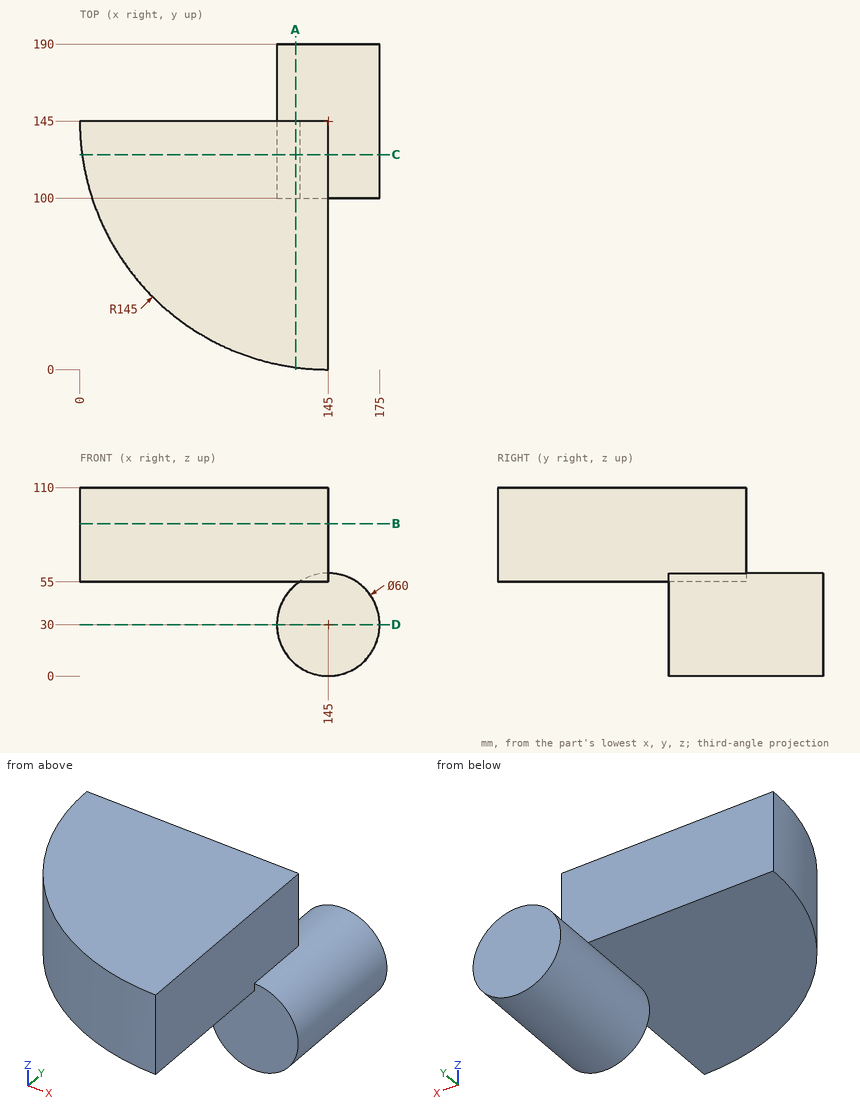
Part print with two shaded views. Sizes in mm from the minimum x, y, z corner. Coordinates: 2 decimals unless noted, no trailing zeros. Write each loop counter-clockwise with the first axis right and the second up, starting at its lowest first coordinate (ties: lowest second). Pieces come first, ordered by that corner, then holes. Notation, with made-up numbers: M -30,65.5 L -13,65.5 A30 ccw -13,88.5 Z; hole C -36,61 d4. An arc over 180 degrees is marked long. Return JSON: item names as keys, results as strings.
Item 1: Probe line 1 (Z direction, x = 124, y = 48); line 2 (Y direction, x = 122, z = 33); line 3 (Z direction, x = 127, y = 118). List the from-to ranges inside material, lowest first. Write a range as from..to.
Findings below:
{"line 1": "z = 55..110", "line 2": "y = 100..190", "line 3": "z = 6..54, 55..110"}
Item 2: Slice it at D-D, the plane z = 30. Write the cut outline in (x, y).
Findings below:
{"outline": "M 115,100 L 175,100 L 175,190 L 115,190 Z"}
Item 3: Drop flat-ended pins along their axis: pin 1 Ø10 at (x, z) = (135.5, 23.5) entering from -Y; pin 2 Ø1.5 at (x, y) = (87.5, 145.5) entering from -Z; pin 3 Ø2 at (x, y) = (32, 146.5) entering from +Z; pin 4 Ø1 at (y, z) = (111, 31) entering from +X. Give the stop position or say it passes through.
Findings below:
{"pin 1": "stops at y = 100", "pin 2": "stops at z = 55", "pin 3": "passes through", "pin 4": "stops at x = 175"}
Item 4: Slice it at C-C, the plane y = 125.5. Write the cut outline in (x, z), and give its area (3 significant figures).
Findings below:
{"outline": "M 1.32,55 L 128.42,55 A30 ccw long 145,60 L 145,110 L 1.32,110 Z", "area": "10,700 mm2"}
Item 5: Slice it at B-B, the plane z = 89. Write the cut outline in (x, y), and give its area (3 significant figures).
Findings below:
{"outline": "M 0,145 A145 ccw 145,0 L 145,145 Z", "area": "16,500 mm2"}
Item 6: Slice it at A-A, the plane x = 126. Write the cut outline in (y, z).
Findings below:
{"outline": "M 1.25,55 L 145,55 L 145,110 L 1.25,110 Z; M 100,6.78 L 190,6.78 L 190,53.22 L 100,53.22 Z"}
